```python
from build123d import *

# Parameters (mm, degrees)
F0_R     = 3.175
F1_DEPTH = 12.7
F2_SIZE  = 1.27
F3_R     = 6.35
F4_DEPTH = 25.4
F5_W     = 101.6
F5_H     = 101.6
F5_R     = 6.35
F6_DEPTH = 6.35


with BuildPart() as f1:
    # F0 (on Right) → F1 (new body)
    with BuildSketch(Plane.YZ):
        Circle(F0_R)
    extrude(amount=F1_DEPTH)

    # F2
    f2_edges = [f1.edges().sort_by_distance(p)[0] for p in [
        (0, -3.175, 0),
    ]]
    chamfer(f2_edges, length=F2_SIZE)

    # F3 (on face) → F4 (join)
    with BuildSketch(Plane.YZ.offset(12.7)):
        Circle(F3_R)
    extrude(amount=F4_DEPTH)

    # F5 (on face) → F6 (join)
    with BuildSketch(Plane.YZ.offset(38.1)):
        Rectangle(F5_W, F5_H)
        Circle(F5_R, mode=Mode.SUBTRACT)
        Circle(F5_R)
    extrude(amount=F6_DEPTH)


solid = f1.part
```
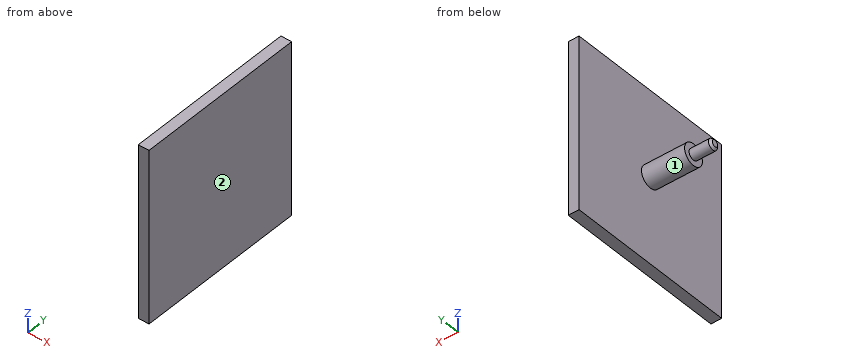
Build history of the part. All positions in model axes, mm. Face numbers are marked on the shaded views. A direction names the side the tool comes from. Give positions to 0.01 mm unless a question says otherwise; leave off trailing zeros. Order: outer loops, then holes, each group sorted by start corner. A loop starts at its lowest first (then second) coordinate and runs counter-clockwise, first axis right, second up. Notation, with made-up numbers: M 46,-2 L 75,-2 A26 cw 75,13 Z; hole C -7,-12 d1. An arc over 180 degrees is marked long. Return JSON: item names as keys, results as strings.
Q1. Band-saw the part on D-D (z = -40). Give the cut face in (x, y), then the cut area to 3 significant figures.
Answer list:
{"outline": "M 38.1,-50.8 L 44.45,-50.8 L 44.45,50.8 L 38.1,50.8 Z", "area": "645 mm^2"}
Q2. Band-saw the part on C-C (x = 36). Give the cut face in (y, z).
Answer list:
{"outline": "C 0,0 d12.7"}
Q3. 3-axis set-ups, long thin cutter, end or side, ignore diameter. For the marked faces 1 and 2: which of +Z, -Z, +X, -X, +Y, -Y reach the whole face in a straight line?
Answer list:
{"face 1": "-X", "face 2": "+Z, -Z, +X, +Y, -Y"}
Q4. Flat gauge pins, fed straight in: pin 1 (4 mm diameter, centred on y = 15, z = 32, fed in from -X); pin 2 (8 mm diameter, centred on x = 15.5, y = 4.5, fed in from -Z). Where does each tip first touch, or does it go through?
Answer list:
{"pin 1": "stops at x = 38.1", "pin 2": "stops at z = -6.33"}
Q5. Band-saw the part on A-A (z = 0). Give the cut face in (x, y) (3 decimals), then the cut area to 3 significant figures.
Answer list:
{"outline": "M 0,-1.905 L 1.27,-3.175 L 12.7,-3.175 L 12.7,-6.35 L 38.1,-6.35 L 38.1,-50.8 L 44.45,-50.8 L 44.45,50.8 L 38.1,50.8 L 38.1,6.35 L 12.7,6.35 L 12.7,3.175 L 1.27,3.175 L 0,1.905 Z", "area": "1,050 mm^2"}
Q6. Wall check: probe 1 along X at (y, z) = (24, -17.5); probe 2 along Z at (x, y) = (20, 0.5); probe 3 along Y at (x, z) = (26.5, -5). Give the ranges that are in metal, low to high. Write a range as from..to.
Answer list:
{"probe 1": "x = 38.1..44.45", "probe 2": "z = -6.33..6.33", "probe 3": "y = -3.91..3.91"}
